```python
from build123d import *

# Parameters (mm, degrees)
ESQUISSE1_W        = 9
ESQUISSE1_H        = 9
BOSS_EXTRU_1_DEPTH = 50
BOSS_EXTRU_3_START = -1.45
ESQUISSE2_R        = 2
BOSS_EXTRU_3_DEPTH = 6.1


with BuildPart() as part:
    # Esquisse1 → Boss.-Extru.1 (new body)
    with BuildSketch(Plane.XY):
        Rectangle(ESQUISSE1_W, ESQUISSE1_H)
    extrude(amount=BOSS_EXTRU_1_DEPTH)

    # Esquisse2 → Boss.-Extru.3 (add)
    with BuildSketch(Plane(origin=(4.5, 0, 0), x_dir=(0, 0, -1), z_dir=(1, 0, 0)).offset(BOSS_EXTRU_3_START)):
        with BuildLine():
            Line((-50, 4.5), (-58.080541819, 4.5))
            ThreePointArc((-58.080541819, 4.5), (-58.982154324, 2.376383494), (-59.29, 0.089927018))
            ThreePointArc((-59.29, 0.089927018), (-58.953679263, -2.297932577), (-57.970885209, -4.5))
            Line((-57.970885209, -4.5), (-50, -4.5))
            Line((-50, -4.5), (-50, 4.5))
        make_face()
        with Locations(Location((-54.645, 0, 0), (0, 0, 90))):
            Circle(ESQUISSE2_R, mode=Mode.SUBTRACT)
    extrude(amount=-BOSS_EXTRU_3_DEPTH)


solid = part.part
```
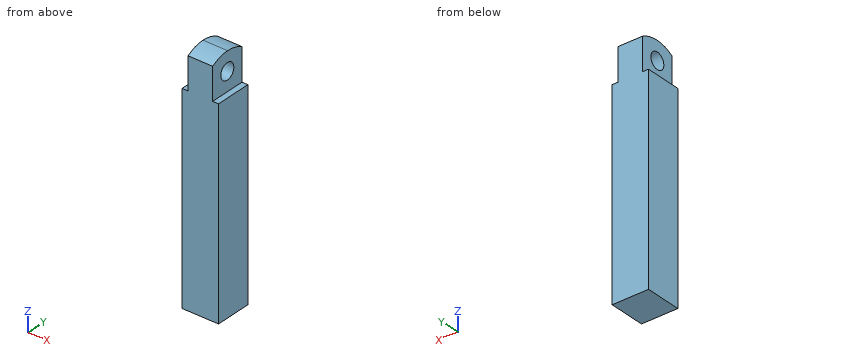
For this review, take the finished solid that the model builds, in its own axes (mm). Coordinates: 2 decimals unless noted, no trailing zeros. Order: outer loops, then holes, each group sorted by start corner. A loop starts at its lowest first (then second) coordinate and runs counter-clockwise, first axis right, second up. Notation, with made-up numbers: (67.25, 15.5) -> (79.25, 15.5) arc R25 cw to (79.25, 51.5) -> close; hole circle Ø8 at (-35, 68). An arc over 180 degrees is marked (long way). Answer as CSV lines item,"result".
Q1. Clearance check with flat-ended pins moving along their axes: pin 1 Ø0.7 at (x, y) = (-3.5, 2) entering from +Z; pin 2 Ø4.5 at (y, z) = (1.5, 55.5) entering from +X; pin 3 Ø2.5 at (y, z) = (-2, 54.5) entering from -X. State where each tip first meets the part, or that it passes through.
Model answer:
pin 1,"stops at z = 50"
pin 2,"stops at x = 3.05"
pin 3,"stops at x = -3.05"
Q2. Wall thickness on line 1 along Z through (x, y) = (-1.5, 0) (3 decimals); line 2 along Z through (x, y) = (-4, -1.75); line 3 along Y through (x, z) = (2.5, 54.5): over which ranges is each line inside the solid? List them lowest first. Write a range as [from, to].
Model answer:
line 1,"z = [0, 52.645], [56.645, 59.29]"
line 2,"z = [0, 50]"
line 3,"y = [-4.5, -1.99], [1.99, 4.5]"
Q3. We need section B-B (x = -1.75). State the section outline as (y, z) points (3 decimals).
Model answer:
outline,"(-4.5, 0) -> (4.5, 0) -> (4.5, 58.081) arc R8.645 ccw to (-4.5, 57.971) -> close; hole circle Ø4 at (0, 54.645)"
Q4. We need section C-C (y = -3.5). State the section outline as (x, z) points.
Model answer:
outline,"(-4.5, 0) -> (4.5, 0) -> (4.5, 50) -> (3.05, 50) -> (3.05, 58.51) -> (-3.05, 58.51) -> (-3.05, 50) -> (-4.5, 50) -> close"
Q5. We need section A-A (y = -1.25). State the section outline as (x, z) points, plus the area to 3 significant figures.
Model answer:
outline,"(-4.5, 0) -> (4.5, 0) -> (4.5, 50) -> (3.05, 50) -> (3.05, 53.08) -> (-3.05, 53.08) -> (-3.05, 50) -> (-4.5, 50) -> close; (-3.05, 56.21) -> (3.05, 56.21) -> (3.05, 59.19) -> (-3.05, 59.19) -> close"
area,"487 mm2"
Q6. We need section D-D (y = 3.5). State the section outline as (x, z) points.
Model answer:
outline,"(-4.5, 0) -> (4.5, 0) -> (4.5, 50) -> (3.05, 50) -> (3.05, 58.59) -> (-3.05, 58.59) -> (-3.05, 50) -> (-4.5, 50) -> close"
